CAD build for the part. Positions are in the model's coordinates, mm. A direction names the side the tool comes from. Give positions to 0.01 mm unless a question says otherwise; leave off trailing zeros. Write each loop counter-clockwise with the first axis right and the second up, starting at its lowest first coordinate (ties: lowest second). Pieces come first, ordered by that corner, then holes. Notation, with made-up numbers: M 48.5,59 L 98.5,59 A28 cw 98.5,91 Z; hole C 52.25,40 d11. An arc over 180 degrees is marked long. One line per question, with ' | ' between items. Start each with the question number.
1. Cut at D-D, the plane x = 13. Write the cut outline in (y, z), then the cut area to 3 significant figures.
2. Cut at A-A, the plane y = 0. Write the cut outline in (x, z).
3. Cut at B-B, the plane x = 0. Write the cut outline in (y, z).
4. Wall check: L1, parallel to X at y = 18, z = 3.75; L2, parallel to X at y = 22, z = -1.75; L3, parallel to Z at x = -19.5, y = 27. Give the ranges that are in metal, low to high.
5. Cut at C-C, the plane z = 7.5. Write the cut outline in (x, y).
6. Flat gauge pins, fed straight in: pin 1 (3.5 mm diameter, centred on x = -24.75, y = -24.75, fed in from +Z); pin 2 (1.3 mm diameter, centred on x = 31, y = -15, fed in from -Z); pin 3 (5.5 mm diameter, centred on x = 18.65, y = -29.02, fed in from -Z); pin 4 (3 mm diameter, centred on y = -27.5, z = 4, fed in from -X). Where does each tip first touch, or does it go through?
7. Pull direction Y, two halves, no side cores. Call faces 5 (the face through (40, 0, 2)), 6 (the face through (31.95, 4.88, -2.54)), 7 (the face through (-35.72, 35.49, 1.9)), 8 (the face through (25.672, 26.523, 6.566)): released by +Y, released by -Y, zero draft, split by the parting line, or undercut.
8. Which spindle directions (+Z, -Z, +X, -X, +Y, -Y) get a long thin tool onto all of the face, cutting with end or side? Do faces 1 (the face through (-27.44, 20.87, -2.54)), 2 (the face through (35.72, -35.49, 1.9)), 3 (the face through (15.043, 28.922, 4.437)), 4 (the face through (26, -23, 4.2)). Say none if no direction does.
Autodesk Inventor part; units mm, degrees
ref_plane "YZ Plane" through (0, 0, 0) normal (1, 0, 0) x (0, 1, 0)
ref_plane "XZ Plane" through (0, 0, 0) normal (0, 1, 0) x (-1, 0, 0)
ref_plane "XY Plane" through (0, 0, 0) normal (0, 0, 1) x (1, 0, 0)
sketch "스케치1" plane through (0, 0, 0) normal (0, 0, 1) x (1, 0, 0)
  line L0 (-25, -30) -> (25, -30) construction
  line L1 (30, -25) -> (30, 25) construction
  line L2 (25, 30) -> (-25, 30) construction
  line L3 (-30, 25) -> (-30, -25) construction
  line L4 (-30, -30) -> (30, 30) construction
  line L5 (30, -30) -> (-30, 30) construction
  arc A0 (-25, 30) -> (-30, 25) centre (-25, 25) ccw
  arc A1 (30, 25) -> (25, 30) centre (25, 25) ccw
  arc A2 (25, -30) -> (30, -25) centre (25, -25) ccw
  arc A3 (-30, -25) -> (-25, -30) centre (-25, -25) ccw
  circle A4 centre (0, 0) radius 7.5
  circle A5 centre (0, 0) radius 35 construction
  circle A6 centre (-24.7487, 24.7487) radius 2
  circle A7 centre (-24.7487, -24.7487) radius 2
  circle A8 centre (24.7487, -24.7487) radius 2
  circle A9 centre (24.7487, 24.7487) radius 2
  circle A10 centre (0, 0) radius 32.6
  circle A11 centre (0, 0) radius 25 construction
  line L6 (-25, 40) -> (25, 40)
  arc A12 (40, 25) -> (25, 40) centre (25, 25) ccw
  line L7 (40, 25) -> (40, -25)
  arc A13 (25, -40) -> (40, -25) centre (25, -25) ccw
  line L8 (25, -40) -> (-25, -40)
  arc A14 (-40, -25) -> (-25, -40) centre (-25, -25) ccw
  line L9 (-40, -25) -> (-40, 25)
  arc A15 (-25, 40) -> (-40, 25) centre (-25, 25) ccw
  dimension "d4" = 70
  dimension "d0" = 60
  dimension "d1" = 60
  dimension "d2" = 5
  dimension "d3" = 15
  dimension "d5" = 4
  dimension "d8" = 360
  dimension "d10" = 65.2
  dimension "d11" = 50
  dimension "d12" = 10
extrude "돌출1" add sketch "스케치1" along normal blind 9 contours L6 A12 L7 A13 L8 A14 L9 A15
sketch "스케치2" plane through (0, 0, 0) normal (0, 0, -1) x (-1, 0, 0)
  line L0 (25, -40) -> (-25, -40)
  arc A0 (25, -40) -> (40, -25) centre (25, -25) ccw
  line L1 (40, 25) -> (40, -25)
  arc A1 (40, 25) -> (25, 40) centre (25, 25) ccw
  line L2 (-25, 40) -> (25, 40)
  arc A2 (-25, 40) -> (-40, 25) centre (-25, 25) ccw
  line L3 (-40, -25) -> (-40, 25)
  arc A3 (-40, -25) -> (-25, -40) centre (-25, -25) ccw
  circle A4 centre (0, 0) radius 32.6 construction
  circle A5 centre (-24.7487, 24.7487) radius 2
  circle A6 centre (-24.7487, -24.7487) radius 2
  circle A7 centre (24.7487, -24.7487) radius 2
  circle A8 centre (24.7487, 24.7487) radius 2
  circle A9 centre (0, 0) radius 29
  dimension "d15" = 58
extrude "돌출2" add sketch "스케치2" along normal blind 5 contours L0 A3 L3 A2 L2 A1 L1 A0 | A5 | A6 | A7 | A8
sketch "스케치9" plane through (0, 0, 0) normal (0, 0, 1) x (1, 0, 0)
  circle A0 centre (-24.7487, 24.7487) radius 2
  line L0 (-28.9057, 24.7487) -> (-26.8272, 28.3487)
  line L1 (-26.8272, 28.3487) -> (-22.6703, 28.3487)
  line L2 (-22.6703, 28.3487) -> (-20.5918, 24.7487)
  line L3 (-20.5918, 24.7487) -> (-22.6703, 21.1487)
  line L4 (-22.6703, 21.1487) -> (-26.8272, 21.1487)
  line L5 (-26.8272, 21.1487) -> (-28.9057, 24.7487)
  line L6 (-28.9057, 24.7487) -> (-28.9057, 15.0739)
  circle A1 centre (0, 0) radius 32.6
  line L7 (-22.6703, 28.3487) -> (-16.0969, 28.3487)
  point P0 (-20.7972, 25.1045)
  point P1 (-24.8091, 21.1487)
  dimension "d27" = 7.2
extrude "돌출4" cut sketch "스케치9" along normal blind 4.2 contours L0 L1 L2 A1 L4 L5 | L5 L4 A1 L6 | L7 A1 L2 | A1 L2 L3 L4 picked at (-21.824, 23.2537)
mirror "미러1" about plane through (0, 0, 0) normal (0, 1, 0) of "돌출4"
mirror "미러2" about plane through (0, 0, 0) normal (1, 0, 0) of "돌출4", "미러1"
sketch "스케치10" plane through (0, 0, -5) normal (0, 0, -1) x (-1, 0, 0)
  circle A0 centre (0, 0) radius 32.5 construction
  circle A1 centre (0, -34.5) radius 2 construction
  circle A2 centre (0, -34.5) radius 2.2
  dimension "d30" = 65
  dimension "d31" = 4
  dimension "d32" = 0.2
extrude "돌출5" cut sketch "스케치10" against normal blind 5
pattern_circular "원형 패턴1" count 11 over 360 about axis through (0, 0, 0) along (0, 0, -1) of "돌출5"
properties part number "사이클로이드 기어 하우징"
Here are the results:
1) outline: M -40,-5 L -25.92,-5 L -25.92,0 L -29.9,0 L -29.9,9 L -40,9 Z; M 25.92,-5 L 40,-5 L 40,9 L 29.9,9 L 29.9,0 L 25.92,0 Z | area: 323 mm^2
2) outline: M -40,-5 L -29,-5 L -29,0 L -32.6,0 L -32.6,9 L -40,9 Z; M 29,-5 L 40,-5 L 40,9 L 32.6,9 L 32.6,0 L 29,0 Z
3) outline: M -40,-5 L -36.7,-5 L -36.7,0 L -32.6,0 L -32.6,9 L -40,9 Z; M -32.3,-5 L -29,-5 L -29,0 L -32.3,0 Z; M 29,-5 L 40,-5 L 40,9 L 32.6,9 L 32.6,0 L 29,0 Z
4) L1: -40 to -28.91, 28.91 to 40 | L2: -40 to -28.19, -23.95 to -18.89, 18.89 to 23.95, 28.19 to 40 | L3: -5 to 0, 4.2 to 9
5) outline: M -40,-25 A15 ccw -25,-40 L 25,-40 A15 ccw 40,-25 L 40,25 A15 ccw 25,40 L -25,40 A15 ccw -40,25 Z; hole C 0,0 d65.2; hole C -24.75,-24.75 d4; hole C -24.75,24.75 d4; hole C 24.75,-24.75 d4; hole C 24.75,24.75 d4
6) pin 1: z = 0 | pin 2: z = 0 | pin 3: z = -5 | pin 4: x = -39.97
7) face 5: zero draft | face 6: undercut | face 7: released by +Y | face 8: undercut
8) face 1: -Z | face 2: +Z, -Z, +X, -Y | face 3: +Z | face 4: none
